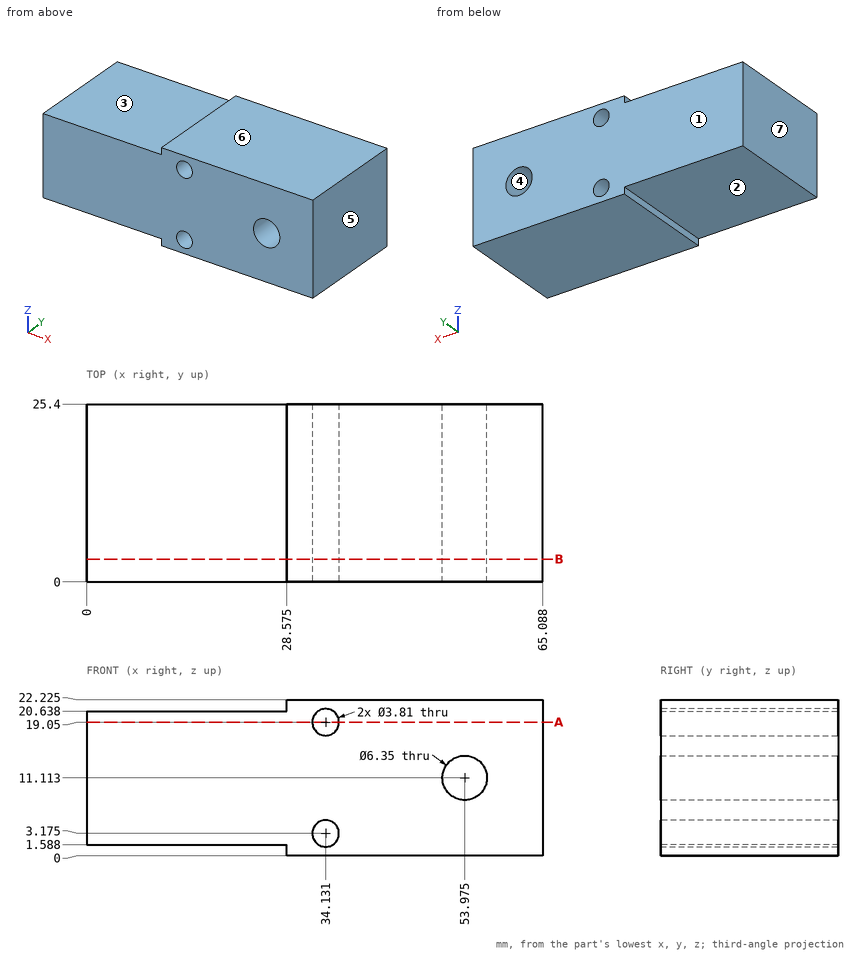
Geometry: see drawing. Coordinates: mm, zero at the bounding-box minimum. A direction names the side the tool comes from. Coordinates: 2 decimals unless noted, no trailing zeros. Loops run counter-clockwise (first coordinate to the right, second up) from the corner with the lowest first, then second, coordinate; pieces in that order, holes last. Notation, with made-up numbers: (83.5, 60.25) -> (112.5, 60.25) arc R30 cw to (112.5, 96.25) -> close; hole circle Ø6 at (88.5, -2). An arc over 180 degrees is marked (long way). Use a Markdown table: item, result.
1) Material intervals for line 1 along X through (y, z) = (15, 3) (1 decimal); line 2 along Z through (x, y) = (28.5, 23); line 3 along X through (y, z) = (4, 10), sorted ascending. Write a range as from..to.
Results found:
| item | result |
|---|---|
| line 1 | x = 0..32.2, 36..65.1 |
| line 2 | z = 1.59..20.64 |
| line 3 | x = 0..51, 56.95..65.09 |
2) Cut plane A-A (z = 19.05). Return the cut outline in (x, y).
Results found:
| item | result |
|---|---|
| outline | (0, 0) -> (32.23, 0) -> (32.23, 25.4) -> (0, 25.4) -> close; (36.04, 0) -> (65.09, 0) -> (65.09, 25.4) -> (36.04, 25.4) -> close |
3) Pull-direction query (X, two-part tool) for the marked faces 4, 5, 6 and 7; classes: released by +X, released by -X, zero draft, split by the parting line, or undercut.
Results found:
| item | result |
|---|---|
| face 4 | undercut |
| face 5 | released by +X |
| face 6 | zero draft |
| face 7 | released by -X |
4) Access query for the marked faces 1, 2 and 3. Directions: +Z, -Z, +X, -X, +Y, -Y. A direction counts if a zero-diameter tool reaches every point of the face in a straight line with its end or side. Return the directions, or none.
Results found:
| item | result |
|---|---|
| face 1 | +Z, -Z, +X, -X, +Y |
| face 2 | -Z, -X, +Y, -Y |
| face 3 | +Z, -X, +Y, -Y |
5) Cut plane B-B (y = 3.25). Give the number of separate pieces and of enclosed holes in the cut face, then the cut area to 3 significant figures.
Results found:
| item | result |
|---|---|
| separate pieces | 1 |
| enclosed holes | 3 |
| area | 1,300 mm2 |
6) Contact query for flat-ended pins moving along their axis: pin 1 (12.5 mm diameter, centred on x = 8, y = 7, fed in from -Z); pin 2 (12 mm diameter, centred on x = 26.5, y = 2.5, fed in from +Z) (1 decimal); pin 3 (4 mm diameter, centred on x = 53.97, z = 11.11, fed in from +Y); pin 4 (4 mm diameter, centred on x = 11, y = 11.5, fed in from +Z). Output: stop coordinate, or through.
Results found:
| item | result |
|---|---|
| pin 1 | stops at z = 1.59 |
| pin 2 | stops at z = 22.2 |
| pin 3 | passes through |
| pin 4 | stops at z = 20.64 |
